```python
from build123d import *

# Parameters (mm, degrees)
BOSS_EXTRUDE1_DEPTH = 32.5
BOSS_EXTRUDE2_DEPTH = 2.5
SKETCH3_W           = 15
SKETCH3_H           = 45
BOSS_EXTRUDE3_DEPTH = 1
SKETCH4_W           = 25
SKETCH4_H           = 55
BOSS_EXTRUDE4_DEPTH = 1


with BuildPart() as part:
    # Sketch1 → Boss-Extrude1 (new, symmetric)
    with BuildSketch(Plane.XY):
        with BuildLine():
            Line((5, 0), (140, 0))
            ThreePointArc((140, 0), (143.535533906, 1.464466094), (145, 5))
            Line((145, 5), (145, 35))
            ThreePointArc((145, 35), (143.535533906, 38.535533906), (140, 40))
            Line((140, 40), (10, 40))
            Line((10, 40), (10, 37.5))
            Line((10, 37.5), (140, 37.5))
            ThreePointArc((140, 37.5), (141.767766953, 36.767766953), (142.5, 35))
            Line((142.5, 35), (142.5, 5))
            ThreePointArc((142.5, 5), (141.767766953, 3.232233047), (140, 2.5))
            Line((140, 2.5), (5, 2.5))
            ThreePointArc((5, 2.5), (3.232233047, 3.232233047), (2.5, 5))
            Line((2.5, 5), (2.5, 40))
            ThreePointArc((2.5, 40), (3.232233047, 41.767766953), (5, 42.5))
            Line((5, 42.5), (40, 42.5))
            Line((40, 42.5), (40, 45))
            Line((40, 45), (5, 45))
            ThreePointArc((5, 45), (1.464466094, 43.535533906), (0, 40))
            Line((0, 40), (0, 5))
            ThreePointArc((0, 5), (1.464466094, 1.464466094), (5, 0))
        make_face()
    extrude(amount=BOSS_EXTRUDE1_DEPTH, both=True)

    # Sketch2 → Boss-Extrude2 (add)
    with BuildSketch(Plane.XY.offset(32.5)):
        with BuildLine():
            Line((0, 40), (0, 5))
            ThreePointArc((0, 5), (1.464466094, 1.464466094), (5, 0))
            Line((5, 0), (140, 0))
            ThreePointArc((140, 0), (143.535533906, 1.464466094), (145, 5))
            Line((145, 5), (145, 35))
            ThreePointArc((145, 35), (143.535533906, 38.535533906), (140, 40))
            Line((140, 40), (0, 40))
        make_face()
    boss_extrude2 = extrude(amount=-BOSS_EXTRUDE2_DEPTH)

    # Mirror1: Boss-Extrude2 across plane
    add(boss_extrude2.mirror(Plane.XY))

    # Sketch3 → Boss-Extrude3 (add)
    with BuildSketch(Plane(origin=(0, 40, 0), x_dir=(1, 0, 0), z_dir=(0, 1, 0))):
        with Locations((37.5, 0)):
            Rectangle(SKETCH3_W, SKETCH3_H)
    extrude(amount=BOSS_EXTRUDE3_DEPTH)

    # Sketch4 → Boss-Extrude4 (add)
    with BuildSketch(Plane.XZ):
        with Locations((22.5, 0)):
            Rectangle(SKETCH4_W, SKETCH4_H)
        with Locations((122.5, 0)):
            Rectangle(SKETCH4_W, SKETCH4_H)
    extrude(amount=BOSS_EXTRUDE4_DEPTH)


solid = part.part
```
Work out the finished part from the listing and answer in its coordinate system (mm). A direction names the side the tool comes from. Give positions to 0.01 mm unless a question says otherwise; leave off trailing zeros. Write each loop counter-clockwise with the first axis right and the second up, starting at its lowest first coordinate (ties: lowest second). Pieces come first, ordered by that corner, then holes. Notation, with made-up numbers: (30.25, 52) -> (63.25, 52) arc R4 ccw to (63.25, 57) -> close; hole circle Ø1 at (53.5, 83). An arc over 180 degrees is marked (long way). Write each question's results on one line, items separated by ' | '.
1. Find section B-B on y = 15. Determine the outline of the cut face in (x, z), and give its area (4 significant figures).
Data:
outline: (0, -32.5) -> (145, -32.5) -> (145, 32.5) -> (0, 32.5) -> close; hole (2.5, -30) -> (142.5, -30) -> (142.5, 30) -> (2.5, 30) -> close | area: 1,025 mm^2
2. Straight lines are drawn through the part: L1, parallel to Y at x = 21.5, z = 12; L2, parallel to X at y = 18, z = -17; L3, parallel to Y at x = 117, z = 13.5. For each, find the intervals that lie inside material, in ascending order.
Data:
L1: -1 to 2.5, 37.5 to 40, 42.5 to 45 | L2: 0 to 2.5, 142.5 to 145 | L3: -1 to 2.5, 37.5 to 40
3. Find section D-D on x = 66. Determine the outline of the cut face in (y, z), and give its area (3 significant figures).
Data:
outline: (0, -32.5) -> (40, -32.5) -> (40, 32.5) -> (0, 32.5) -> close; hole (2.5, -30) -> (37.5, -30) -> (37.5, 30) -> (2.5, 30) -> close | area: 500 mm^2
4. Find section A-A on x = 27. Determine the outline of the cut face in (y, z).
Data:
outline: (-1, -27.5) -> (0, -27.5) -> (0, -32.5) -> (40, -32.5) -> (40, 32.5) -> (0, 32.5) -> (0, 27.5) -> (-1, 27.5) -> close; (42.5, -32.5) -> (45, -32.5) -> (45, 32.5) -> (42.5, 32.5) -> close; hole (2.5, -30) -> (37.5, -30) -> (37.5, 30) -> (2.5, 30) -> close
5. Determine the mould class of faces 1 (the cylindrical face through (2, 44, 0)), 2 (the flat face through (71, 23, -32.5)), 3 (the flat face through (74, 37.5, 0)) for opening direction Y: +Y half, -Y half, draft (parallel to the pull), parting line (faces both ways), or undercut.
Data:
face 1: +Y half | face 2: draft | face 3: undercut
6. Each of these flat-tipped pins is pushed along its axis until it touches: pin 1 Ø0.5 at (y, z) = (-0.5, -10) entering from +X; pin 2 Ø6 at (x, z) = (107, 18.5) entering from +Y; pin 3 Ø0.8 at (y, z) = (-0.5, 7.5) entering from -X. Where does it stop, or does it pass through?
Data:
pin 1: x = 135 | pin 2: y = 40 | pin 3: x = 10
7. A tool of negligible diameter and unlimited length cuts with its end or side. For faces 4 (the flat face through (40, 44, 0)), 5 (the flat face through (37, 41, 0)), 6 (the flat face through (142.5, 20, 0)), from which of +Z, -Z, +X, -X, +Y, -Y can it reach the whole face along a straight path? Write none if from no direction.
Data:
face 4: +Z, -Z, +X, +Y | face 5: +Z, -Z, +X | face 6: none
